```python
from build123d import *

# Parameters (mm, degrees)
SKETCH1_W           = 127
SKETCH1_H           = 44.45
BOSS_EXTRUDE1_DEPTH = 5.08
CUT_EXTRUDE1_DEPTH  = 0.9652


with BuildPart() as part:
    # Sketch1 → Boss-Extrude1 (new body)
    with BuildSketch(Plane.XY):
        Rectangle(SKETCH1_W, SKETCH1_H)
    extrude(amount=BOSS_EXTRUDE1_DEPTH)

    # Sketch3 → Cut-Extrude1 (cut)
    with BuildSketch(Plane(origin=(0, 0, 0), x_dir=(-1, 0, 0), z_dir=(0, 0, -1))):
        with BuildLine():
            Line((-63.5, 14.9606), (-34.365536726, 14.9606))
            ThreePointArc((-34.365536726, 14.9606), (-31.071645561, 14.039483955), (-28.733362586, 11.543365668))
            ThreePointArc((-28.733362586, 11.543365668), (-25.908, 0), (-28.733362586, -11.543365668))
            ThreePointArc((-28.733362586, -11.543365668), (-31.071645561, -14.039483955), (-34.365536726, -14.9606))
            Line((-34.365536726, -14.9606), (-63.5, -14.9606))
            Line((-63.5, -14.9606), (-63.5, 14.9606))
        make_face()
    extrude(amount=-CUT_EXTRUDE1_DEPTH, mode=Mode.SUBTRACT)


solid = part.part
```
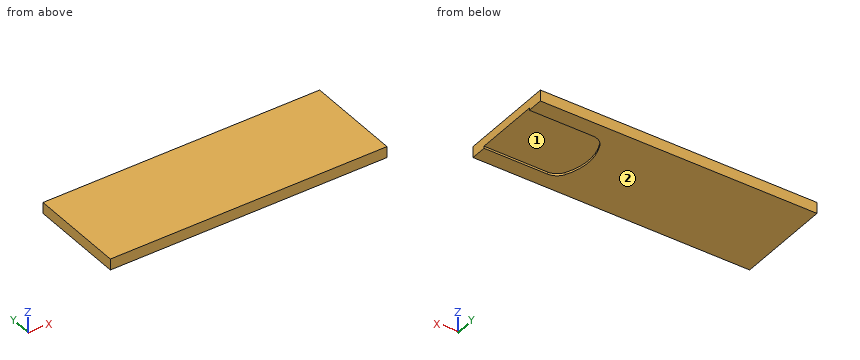
Check sheet for the modelled part. Datum: model origin and axes. Units: mm. Face numbers are marked on the shaded views. Round coordinates to 2 decimals unless told otherwise and drop trailing zeros. Loops run counter-clockwise (first coordinate to the right, second up) from the corner with the lowest first, then second, coordinate; pieces in that order, holes last. Notation, with made-up numbers: M 55.25,-38 L 89.25,-38 A23 ccw 89.25,-17 Z; hole C -35,72.25 d11. An arc over 180 degrees is marked long. Answer as a JSON object with one key per item and string values.
1. Section check D-D (y = -1.5). Record the boundary of the cut face in (x, z), plus the area to 3 significant figures.
Reply:
{"outline": "M -63.5,0 L 25.95,0 L 25.95,0.97 L 63.5,0.97 L 63.5,5.08 L -63.5,5.08 Z", "area": "609 mm²"}
2. Scan lines: line 1 (Y direction, x = 49.5, z = 0.65) (3 decimals); line 2 (Z direction, x = 42, y = 7.5); line 3 (X direction, y = 13.5, z = 0.45). Record each from-to range of solid material in increasing order.
Reply:
{"line 1": "y = -22.225 to -14.961, 14.961 to 22.225", "line 2": "z = 0.97 to 5.08", "line 3": "x = -63.5 to 30.31"}
3. Section check B-B (y = 8.5). Record the boundary of the cut face in (x, z).
Reply:
{"outline": "M -63.5,0 L 27.4,0 L 27.4,0.97 L 63.5,0.97 L 63.5,5.08 L -63.5,5.08 Z"}
4. Section check A-A (x = 55). Record the boundary of the cut face in (y, z) (3 decimals).
Reply:
{"outline": "M -22.225,0 L -14.961,0 L -14.961,0.965 L 14.961,0.965 L 14.961,0 L 22.225,0 L 22.225,5.08 L -22.225,5.08 Z"}
5. Section check C-C (x = 27.5). Record the boundary of the cut face in (y, z) (3 decimals), plus the area to 3 significant figures.
Reply:
{"outline": "M -22.225,0 L -8.778,0 L -8.778,0.965 L 8.778,0.965 L 8.778,0 L 22.225,0 L 22.225,5.08 L -22.225,5.08 Z", "area": "209 mm²"}
6. Gauge pin test, flat ends, axial feed: P1, Ø1, axis at x = -7, y = 3.5, coming from the -Z side; P2, Ø9, axis at x = 45.5, y = 2.5, coming from the -Z side. Record the tip position at first contact, or that the pin passes through.
Reply:
{"P1": "stops at z = 0", "P2": "stops at z = 0.97"}
7. Mould release check, pull along Y, two halves, no side actions. Record for the marked faces 1 and 2: pulls with the +Y half, pulls with the -Y half, needs draft (parallel to the pull), parting line crosses it, or undercut.
Reply:
{"face 1": "undercut", "face 2": "needs draft"}
